from build123d import *

# Parameters (mm, degrees)
SKETCH1_R           = 2
SKETCH1_R_2         = 3
SKETCH1_W           = 13
SKETCH1_H           = 8.25
BOSS_EXTRUDE1_DEPTH = 6.35
FILLET1_R           = 1.5
SKETCH2_W           = 82.327825706
SKETCH2_H           = 14.458254131
CUT_EXTRUDE1_DEPTH  = 51
SKETCH3_W           = 51.5
SKETCH3_H           = 6.35
BOSS_EXTRUDE2_DEPTH = 25


with BuildPart() as part:
    # Sketch1 → Boss-Extrude1 (new body)
    with BuildSketch(Plane(origin=(0, 0, 0), x_dir=(1, 0, 0), z_dir=(0, 1, 0))):
        Polygon((38, 0), (38, 5), (58, 5), (58, 0), (96, 0), (96, 48.5), (89, 58.5), (89, 67.5), (62, 67.5), (62, 56.5), (34, 56.5), (34, 67.5), (7, 67.5), (7, 58.5), (0, 48.5), (0, 0), align=None)
        with Locations(Location((38.5, 40, 0), (0, 0, 270))):
            Circle(SKETCH1_R, mode=Mode.SUBTRACT)
        with Locations(Location((38.5, 22, 0), (0, 0, 270))):
            Circle(SKETCH1_R, mode=Mode.SUBTRACT)
        with Locations(Location((57.5, 22, 0), (0, 0, 90))):
            Circle(SKETCH1_R, mode=Mode.SUBTRACT)
        with Locations(Location((57.5, 40, 0), (0, 0, 90))):
            Circle(SKETCH1_R, mode=Mode.SUBTRACT)
        with Locations(Location((12.5, 61.75, 0), (0, 0, 270))):
            Circle(SKETCH1_R_2, mode=Mode.SUBTRACT)
        with Locations(Location((28, 61.75, 0), (0, 0, 270))):
            Circle(SKETCH1_R_2, mode=Mode.SUBTRACT)
        with Locations(Location((68, 61.75, 0), (0, 0, 90))):
            Circle(SKETCH1_R_2, mode=Mode.SUBTRACT)
        with Locations(Location((83.5, 61.75, 0), (0, 0, 90))):
            Circle(SKETCH1_R_2, mode=Mode.SUBTRACT)
        with Locations((72.5, 18.625)):
            Rectangle(SKETCH1_W, SKETCH1_H, mode=Mode.SUBTRACT)
        with Locations((23.5, 34.875)):
            Rectangle(SKETCH1_W, SKETCH1_H, mode=Mode.SUBTRACT)
        with Locations((23.5, 18.625)):
            Rectangle(SKETCH1_W, SKETCH1_H, mode=Mode.SUBTRACT)
        with Locations((72.5, 34.875)):
            Rectangle(SKETCH1_W, SKETCH1_H, mode=Mode.SUBTRACT)
        with BuildLine():
            Line((2.75, 11.75), (5.75, 11.75))
            ThreePointArc((5.75, 11.75), (7.5, 10), (5.75, 8.25))
            Line((5.75, 8.25), (2.75, 8.25))
            ThreePointArc((2.75, 8.25), (1, 10), (2.75, 11.75))
        make_face(mode=Mode.SUBTRACT)
        with BuildLine():
            Line((93.25, 8.25), (90.25, 8.25))
            ThreePointArc((90.25, 8.25), (88.5, 10), (90.25, 11.75))
            Line((90.25, 11.75), (93.25, 11.75))
            ThreePointArc((93.25, 11.75), (95, 10), (93.25, 8.25))
        make_face(mode=Mode.SUBTRACT)
        with BuildLine():
            Line((93.25, 45.5), (90.25, 45.5))
            ThreePointArc((90.25, 45.5), (88.5, 47.25), (90.25, 49))
            Line((90.25, 49), (93.25, 49))
            ThreePointArc((93.25, 49), (95, 47.25), (93.25, 45.5))
        make_face(mode=Mode.SUBTRACT)
        with BuildLine():
            Line((2.75, 49), (5.75, 49))
            ThreePointArc((5.75, 49), (7.5, 47.25), (5.75, 45.5))
            Line((5.75, 45.5), (2.75, 45.5))
            ThreePointArc((2.75, 45.5), (1, 47.25), (2.75, 49))
        make_face(mode=Mode.SUBTRACT)
    extrude(amount=BOSS_EXTRUDE1_DEPTH)

    # Fillet1
    fillet1_edges = [part.edges().sort_by_distance(p)[0] for p in [
        (0, 3.175, -48.5),
        (7, 3.175, -58.5),
        (7, 3.175, -67.5),
        (34, 3.175, -67.5),
        (34, 3.175, -56.5),
        (62, 3.175, -56.5),
        (62, 3.175, -67.5),
        (89, 3.175, -67.5),
        (89, 3.175, -58.5),
        (96, 3.175, -48.5),
        (96, 3.175, 0),
        (58, 3.175, 0),
        (58, 3.175, -5),
        (38, 3.175, -5),
        (38, 3.175, 0),
        (0, 3.175, 0),
        (17, 3.175, -39),
        (17, 3.175, -30.75),
        (30, 3.175, -30.75),
        (30, 3.175, -39),
        (17, 3.175, -22.75),
        (17, 3.175, -14.5),
        (30, 3.175, -14.5),
        (30, 3.175, -22.75),
        (79, 3.175, -14.5),
        (79, 3.175, -22.75),
        (66, 3.175, -22.75),
        (66, 3.175, -14.5),
        (79, 3.175, -30.75),
        (79, 3.175, -39),
        (66, 3.175, -39),
        (66, 3.175, -30.75),
    ]]
    fillet(fillet1_edges, radius=FILLET1_R)

    # Sketch2 → Cut-Extrude1 (cut)
    with BuildSketch(Plane(origin=(48, 0, 0), x_dir=(0, 0, -1), z_dir=(1, 0, 0))):
        with Locations((33.293792952, 1.315835649)):
            Rectangle(SKETCH2_W, SKETCH2_H)
    extrude(amount=CUT_EXTRUDE1_DEPTH, mode=Mode.SUBTRACT)

    # Sketch3 → Boss-Extrude2 (add)
    with BuildSketch(Plane(origin=(48, 0, 0), x_dir=(0, 0, -1), z_dir=(1, 0, 0))):
        with Locations((30.75, 3.175)):
            Rectangle(SKETCH3_W, SKETCH3_H)
    extrude(amount=BOSS_EXTRUDE2_DEPTH)

    # Mirror1: part across plane


with BuildPart() as part_1:
    add(part.part)
    add(part.part.mirror(Plane(origin=(73, 0, 0), x_dir=(0, 0, 1), z_dir=(1, 0, 0))))


solid = part_1.part
Check sheet for the modelled part. Datum: model origin and axes. Units: mm. A direction names the side the tool comes from. Give positions to 0.01 mm unless a question says otherwise; leave off trailing zeros. Write each loop counter-clockwise with the first axis right and the second up, starting at its lowest first coordinate (ties: lowest second). Pieces come first, ordered by that corner, then holes. Notation, with made-up numbers: (89, 51) -> (106, 51) arc R15 ccw to (106, 62) -> close; hole circle Ø2 at (50.25, 89.5). An arc over 180 degrees is marked (long way). One line per item, written item: value. Start each with the question number.
Item 1: Gauge pin test, flat ends, axial feed: pin 1 (1 mm diameter, centred on x = 103, y = 5, fed in from -Z); pin 2 (1.9 mm diameter, centred on x = 69.5, y = 1.5, fed in from +Z); pin 3 (2.5 mm diameter, centred on x = 38.5, z = -40, fed in from +Y); pin 4 (1.5 mm diameter, centred on x = 3.5, y = 2.5, fed in from -Z). Record the tip position at first contact, or that the pin passes through.
Item 2: Section check C-C on y = 2. State how many separate pieces and enclosed holes the cut face has, then the cut area to 3 significant figures.
Item 3: Section check A-A on z = -10. Record the cut outline in (x, y).
Item 4: Draft check along Z on faces 1 (the flat face through (125, 3, -67.5)), 2 (the flat face through (139, 3, -63)), 3 (the cylindrical face through (10.675, 3.131, -64.131)). Enter one of: +Z half, -Z half, draft (parallel to the pull), parting line (faces both ways), or undercut.
Item 5: Material ranges on probe 1 along Z at (x, y) = (127.5, 4); probe 2 along X at (y, z) = (1.75, -61.75); probe 3 along X at (y, z) = (4.25, -33), recorded low to high. Write a range as from..to.
Item 6: Tool access check on faces 4 (the flat face through (7, 3, -63)), 5 (the flat face through (74, 3, -56.5)), 6 (the flat face through (30, 3, -35)). Record the directions out of +Z, -Z, +X, -X, +Y, -Y that give a thin tool (end or side, any length) a straight path to the whole face; none if there is none.
Item 7: Section check B-B on x = 12.5. Record the cut outline in (y, z).
Item 8: Section check D-D on z = -53. Record the cut outline in (x, y).
Results list:
1. pin 1: z = -56.5
1. pin 2: z = -5
1. pin 3: through
1. pin 4: z = -54.57
2. separate pieces: 1
2. enclosed holes: 16
2. area: 7,780 mm²
3. outline: (0, 0) -> (1, 0) -> (1, 6.35) -> (0, 6.35) -> close; (7.5, 0) -> (138.5, 0) -> (138.5, 6.35) -> (7.5, 6.35) -> close; (145, 0) -> (146, 0) -> (146, 6.35) -> (145, 6.35) -> close
4. face 1: -Z half
4. face 2: draft
4. face 3: undercut
5. probe 1: -67.5..-39, -30.75..-22.75, -14.5..0
5. probe 2: 7..9.5, 15.5..25, 31..34, 112..115, 121..130.5, 136.5..139
5. probe 3: 0..17, 30..116, 129..146
6. face 4: -Z, -X, +Y, -Y
6. face 5: -Z, +Y, -Y
6. face 6: +Y, -Y
7. outline: (0, -67.5) -> (6.35, -67.5) -> (6.35, -64.75) -> (0, -64.75) -> close; (0, -58.75) -> (6.35, -58.75) -> (6.35, 0) -> (0, 0) -> close
8. outline: (3.15, 0) -> (142.85, 0) -> (142.85, 6.35) -> (3.15, 6.35) -> close
